```python
from build123d import *

# Parameters (mm, degrees)
SKETCH_2_W               = 54.99
SKETCH_2_H               = 54.99
EXTRUDE_1_DEPTH          = 2
SKETCH_3_R               = 1.5
CUT_EXTRUDE_1_DEPTH      = 3
MIRROR_2_COPY_1_SKETCH_R = 1.5
MIRROR_2_COPY_1_DEPTH    = 3
SKETCH_4_W               = 18
SKETCH_4_H               = 20
EXTRUDE_2_DEPTH          = 10
SKETCH_5_W               = 18
SKETCH_5_H               = 10.1
EXTRUDE_3_DEPTH          = 10


with BuildPart() as part:
    # Sketch 2 → Extrude 1 (new body)
    with BuildSketch(Plane.XY):
        Rectangle(SKETCH_2_W, SKETCH_2_H)
    extrude(amount=EXTRUDE_1_DEPTH)

    # Sketch 3 → Cut-Extrude 1 (cut, through all)
    with BuildSketch(Plane.XY.offset(2)):
        with Locations((-24.115, -24.115)):
            Circle(SKETCH_3_R)
    cut_extrude_1 = extrude(amount=-CUT_EXTRUDE_1_DEPTH, mode=Mode.SUBTRACT)

    # Mirror 1: Cut-Extrude 1 across plane
    add(cut_extrude_1.mirror(Plane.ZX), mode=Mode.SUBTRACT)

    # Mirror 2: Cut-Extrude 1 across plane
    add(cut_extrude_1.mirror(Plane(origin=(0, 0, 0), x_dir=(0, 0, 1), z_dir=(1, 0, 0))), mode=Mode.SUBTRACT)

    # Mirror 2 copy 1 sketch → Mirror 2 copy 1 (cut, through all)
    with BuildSketch(Plane(origin=(0, 0, 2), x_dir=(-1, 0, 0), z_dir=(0, 0, 1))):
        with Locations((-24.115, -24.115)):
            Circle(MIRROR_2_COPY_1_SKETCH_R)
    extrude(amount=-MIRROR_2_COPY_1_DEPTH, mode=Mode.SUBTRACT)

    # Sketch 4 → Extrude 2 (add)
    with BuildSketch(Plane.XY.offset(2)):
        with Locations((25.995, 7.195)):
            Rectangle(SKETCH_4_W, SKETCH_4_H)
    extrude(amount=EXTRUDE_2_DEPTH)

    # Sketch 5 → Extrude 3 (add)
    with BuildSketch(Plane.XY.offset(2)):
        with Locations((25.995, -12.855)):
            Rectangle(SKETCH_5_W, SKETCH_5_H)
    extrude_3 = extrude(amount=EXTRUDE_3_DEPTH)

    # Mirror 3: Extrude 3 across plane
    add(extrude_3.mirror(Plane(origin=(0, 0, 0), x_dir=(0, 0, 1), z_dir=(1, 0, 0))))


solid = part.part
```
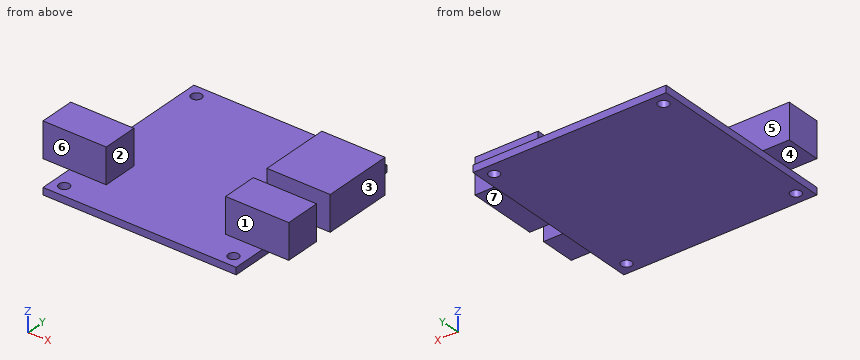
CAD build for the part. Positions are in the model's coordinates, mm. Face numbers are marked on the shaded views. A direction names the side the tool comes from. Round coordinates to 2 decimals unless told otherwise and drop trailing zeros. Order: outer loops, then holes, each group sorted by start corner. A loop starts at its lowest first (then second) coordinate and runs counter-clockwise, first axis right, second up. Notation, with made-up numbers: (-34, 78.5) -> (-28, 78.5) arc R17 ccw to (-28, 87.5) -> close; hole circle Ø2 at (-30, -4.5). An arc over 180 degrees is marked (long way). One line per question, with ' | ' between items.
Q1. Slice it at C-C (y = -12). Write the cut outline in (x, z) (3 decimals).
Completed:
outline: (-34.995, 2) -> (-27.495, 2) -> (-27.495, 0) -> (27.495, 0) -> (27.495, 2) -> (34.995, 2) -> (34.995, 12) -> (16.995, 12) -> (16.995, 2) -> (-16.995, 2) -> (-16.995, 12) -> (-34.995, 12) -> close
Q2. Which spindle directions (+Z, -Z, +X, -X, +Y, -Y) get a long thin tool onto all of the face, cutting with end or side? Do the marked faces 4, 5, 6 and 7. Say none if no direction does.
Completed:
face 4: -Z, -X, +Y, -Y | face 5: +Z, +X, -X, +Y | face 6: +Z, +X, -X, -Y | face 7: -Z, +X, +Y, -Y
Q3. Probe probe 1 along Y at (x, z) = (18.5, 11.25) (3 decimals); probe 2 along Z at (x, y) = (30, -1); probe 3 along X at (y, z) = (-10, 10) (3 decimals). List the from-to ranges inside material, lowest first.
Completed:
probe 1: y = -17.905 to -7.805, -2.805 to 17.195 | probe 2: z = 2 to 12 | probe 3: x = -34.995 to -16.995, 16.995 to 34.995
Q4. Slice it at A-A (x = 30). Write the cut outline in (y, z) (3 decimals), then the cut area to 3 significant figures.
Completed:
outline: (-17.905, 2) -> (-7.805, 2) -> (-7.805, 12) -> (-17.905, 12) -> close; (-2.805, 2) -> (17.195, 2) -> (17.195, 12) -> (-2.805, 12) -> close | area: 301 mm^2
Q5. Drop flat-ended pins along their axis: pin 1 (6 mm diameter, centred on x = -25.5, z = 7.5, fed in from +Y) (3 decimals); pin 2 (8.5 mm diameter, centred on x = 32.5, y = -12.5, fed in from -Z); pin 3 (3 mm diameter, centred on x = 27, z = 8, fed in from -Y) (3 decimals); pin 4 (1.5 mm diameter, centred on x = -10.5, y = -14.5, fed in from -Z). Give the stop position or say it passes through.
Completed:
pin 1: stops at y = -7.805 | pin 2: stops at z = 2 | pin 3: stops at y = -17.905 | pin 4: stops at z = 0
Q6. Slice it at B-B (z = 4.5). Write the cut outline in (x, y) (3 decimals), then the cut area to 3 significant figures.
Completed:
outline: (-34.995, -17.905) -> (-16.995, -17.905) -> (-16.995, -7.805) -> (-34.995, -7.805) -> close; (16.995, -17.905) -> (34.995, -17.905) -> (34.995, -7.805) -> (16.995, -7.805) -> close; (16.995, -2.805) -> (34.995, -2.805) -> (34.995, 17.195) -> (16.995, 17.195) -> close | area: 724 mm^2
Q7. Slice it at D-D (z = 1.25). Write the cut outline in (x, y) (3 decimals).
Completed:
outline: (-27.495, -27.495) -> (27.495, -27.495) -> (27.495, 27.495) -> (-27.495, 27.495) -> close; hole circle Ø3 at (-24.115, -24.115); hole circle Ø3 at (-24.115, 24.115); hole circle Ø3 at (24.115, -24.115); hole circle Ø3 at (24.115, 24.115)
Q8. Two-plate mould, pull along X, no slides. Class the marked faces 1, 2 and 3: released by +X, released by -X, zero draft, split by the parting line, or undercut.
Completed:
face 1: zero draft | face 2: undercut | face 3: released by +X
